Geometry check sheet. Reference: the model listing, model coordinates, mm. Round coordinates to 2 decimals unless told otherwise and drop trailing zeros. Write each loop counter-clockwise with the first axis right and the second up, starting at its lowest first coordinate (ties: lowest second). Pieces come first, ordered by that corner, then holes. Notation, with made-up numbers: (77, 61.25) -> (109, 61.25) arc R22 cw to (109, 68.25) -> close; hole circle Ø7 at (5, -22). An arc over 180 degrees is marked (long way). Use a Markdown table: item, result.
```python
from build123d import *

# Parameters (mm, degrees)
BOSS_EXTRUDE1_DEPTH = 6.35
CHAMFER1_SIZE       = 0.79375
SKETCH16_W          = 3.558466008
SKETCH16_H          = 3.18996611
CUT_EXTRUDE14_DEPTH = 208.663320883
SKETCH21_R          = 0.79375
CUT_EXTRUDE16_DEPTH = 3.175
LPATTERN3_COUNT     = 3
LPATTERN3_PITCH     = 2.032


# Read off the part's stored shape, not the designer's step: Boss-Extrude1
with BuildPart() as part:
    # Boss-Extrude1 outline → Boss-Extrude1 (new body)
    with BuildSketch(Plane.XY):
        with BuildLine():
            Line((22.436796564, 150), (19.069200519, 150))
            ThreePointArc((19.069200519, 150), (17.946668504, 150), (17.946668504, 151.122532015))
            Line((17.946668504, 151.122532015), (17.946668504, 158.877467985))
            ThreePointArc((17.946668504, 158.877467985), (17.946668504, 160), (19.069200519, 160))
            Line((19.069200519, 160), (22.436796564, 160))
            Line((22.436796564, 160), (22.436796564, 170))
            Line((22.436796564, 170), (19.069200519, 170))
            ThreePointArc((19.069200519, 170), (17.946668504, 170), (17.946668504, 171.122532015))
            Line((17.946668504, 171.122532015), (17.946668504, 178.877467985))
            ThreePointArc((17.946668504, 178.877467985), (17.946668504, 180), (19.069200519, 180))
            Line((19.069200519, 180), (22.436796564, 180))
            Line((22.436796564, 180), (22.436796564, 206.35))
            Line((22.436796564, 206.35), (17.436796564, 206.35))
            Line((17.436796564, 206.35), (17.436796564, 201.122532015))
            ThreePointArc((17.436796564, 201.122532015), (17.436796564, 200), (16.314264549, 200))
            Line((16.314264549, 200), (6.35, 200))
            Line((6.35, 200), (6.35, 191.122532015))
            ThreePointArc((6.35, 191.122532015), (6.35, 190), (5.227467985, 190))
            Line((5.227467985, 190), (0, 190))
            Line((0, 190), (0, 180))
            Line((0, 180), (5.227467985, 180))
            ThreePointArc((5.227467985, 180), (6.35, 180), (6.35, 178.877467985))
            Line((6.35, 178.877467985), (6.35, 171.122532015))
            ThreePointArc((6.35, 171.122532015), (6.35, 170), (5.227467985, 170))
            Line((5.227467985, 170), (0, 170))
            Line((0, 170), (0, 160))
            Line((0, 160), (5.227467985, 160))
            ThreePointArc((5.227467985, 160), (6.35, 160), (6.35, 158.877467985))
            Line((6.35, 158.877467985), (6.35, 151.122532015))
            ThreePointArc((6.35, 151.122532015), (6.35, 150), (5.227467985, 150))
            Line((5.227467985, 150), (0, 150))
            Line((0, 150), (0, 140))
            Line((0, 140), (5.227467985, 140))
            ThreePointArc((5.227467985, 140), (6.35, 140), (6.35, 138.877467985))
            Line((6.35, 138.877467985), (6.35, 131.122532015))
            ThreePointArc((6.35, 131.122532015), (6.35, 130), (5.227467985, 130))
            Line((5.227467985, 130), (0, 130))
            Line((0, 130), (0, 120))
            Line((0, 120), (5.227467985, 120))
            ThreePointArc((5.227467985, 120), (6.35, 120), (6.35, 118.877467985))
            Line((6.35, 118.877467985), (6.35, 111.122532015))
            ThreePointArc((6.35, 111.122532015), (6.35, 110), (5.227467985, 110))
            Line((5.227467985, 110), (0, 110))
            Line((0, 110), (0, 100))
            Line((0, 100), (5.227467985, 100))
            ThreePointArc((5.227467985, 100), (6.35, 100), (6.35, 98.877467985))
            Line((6.35, 98.877467985), (6.35, 91.122532015))
            ThreePointArc((6.35, 91.122532015), (6.35, 90), (5.227467985, 90))
            Line((5.227467985, 90), (0, 90))
            Line((0, 90), (0, 80))
            Line((0, 80), (5.227467985, 80))
            ThreePointArc((5.227467985, 80), (6.35, 80), (6.35, 78.877467985))
            Line((6.35, 78.877467985), (6.35, 71.122532015))
            ThreePointArc((6.35, 71.122532015), (6.35, 70), (5.227467985, 70))
            Line((5.227467985, 70), (0, 70))
            Line((0, 70), (0, 60))
            Line((0, 60), (5.227467985, 60))
            ThreePointArc((5.227467985, 60), (6.35, 60), (6.35, 58.877467985))
            Line((6.35, 58.877467985), (6.35, 51.122532015))
            ThreePointArc((6.35, 51.122532015), (6.35, 50), (5.227467985, 50))
            Line((5.227467985, 50), (0, 50))
            Line((0, 50), (0, 40))
            Line((0, 40), (5.227467985, 40))
            ThreePointArc((5.227467985, 40), (6.35, 40), (6.35, 38.877467985))
            Line((6.35, 38.877467985), (6.35, 31.122532015))
            ThreePointArc((6.35, 31.122532015), (6.35, 30), (5.227467985, 30))
            Line((5.227467985, 30), (0, 30))
            Line((0, 30), (0, 20))
            Line((0, 20), (5.227467985, 20))
            ThreePointArc((5.227467985, 20), (6.35, 20), (6.35, 18.877467985))
            Line((6.35, 18.877467985), (6.35, 11.122532015))
            ThreePointArc((6.35, 11.122532015), (6.35, 10), (5.227467985, 10))
            Line((5.227467985, 10), (0, 10))
            Line((0, 10), (0, 0))
            Line((0, 0), (16.314264549, 0))
            ThreePointArc((16.314264549, 0), (17.436796564, 0), (17.436796564, -1.122532015))
            Line((17.436796564, -1.122532015), (17.436796564, -6.35))
            Line((17.436796564, -6.35), (22.436796564, -6.35))
            Line((22.436796564, -6.35), (22.436796564, 10))
            Line((22.436796564, 10), (19.069200519, 10))
            ThreePointArc((19.069200519, 10), (17.946668504, 10), (17.946668504, 11.122532015))
            Line((17.946668504, 11.122532015), (17.946668504, 18.877467985))
            ThreePointArc((17.946668504, 18.877467985), (17.946668504, 20), (19.069200519, 20))
            Line((19.069200519, 20), (22.436796564, 20))
            Line((22.436796564, 20), (22.436796564, 30))
            Line((22.436796564, 30), (19.069200519, 30))
            ThreePointArc((19.069200519, 30), (17.946668504, 30), (17.946668504, 31.122532015))
            Line((17.946668504, 31.122532015), (17.946668504, 38.877467985))
            ThreePointArc((17.946668504, 38.877467985), (17.946668504, 40), (19.069200519, 40))
            Line((19.069200519, 40), (22.436796564, 40))
            Line((22.436796564, 40), (22.436796564, 50))
            Line((22.436796564, 50), (19.069200519, 50))
            ThreePointArc((19.069200519, 50), (17.946668504, 50), (17.946668504, 51.122532015))
            Line((17.946668504, 51.122532015), (17.946668504, 58.877467985))
            ThreePointArc((17.946668504, 58.877467985), (17.946668504, 60), (19.069200519, 60))
            Line((19.069200519, 60), (22.436796564, 60))
            Line((22.436796564, 60), (22.436796564, 70))
            Line((22.436796564, 70), (19.069200519, 70))
            ThreePointArc((19.069200519, 70), (17.946668504, 70), (17.946668504, 71.122532015))
            Line((17.946668504, 71.122532015), (17.946668504, 78.877467985))
            ThreePointArc((17.946668504, 78.877467985), (17.946668504, 80), (19.069200519, 80))
            Line((19.069200519, 80), (22.436796564, 80))
            Line((22.436796564, 80), (22.436796564, 90))
            Line((22.436796564, 90), (19.069200519, 90))
            ThreePointArc((19.069200519, 90), (17.946668504, 90), (17.946668504, 91.122532015))
            Line((17.946668504, 91.122532015), (17.946668504, 98.877467985))
            ThreePointArc((17.946668504, 98.877467985), (17.946668504, 100), (19.069200519, 100))
            Line((19.069200519, 100), (22.436796564, 100))
            Line((22.436796564, 100), (22.436796564, 110))
            Line((22.436796564, 110), (19.069200519, 110))
            ThreePointArc((19.069200519, 110), (17.946668504, 110), (17.946668504, 111.122532015))
            Line((17.946668504, 111.122532015), (17.946668504, 118.877467985))
            ThreePointArc((17.946668504, 118.877467985), (17.946668504, 120), (19.069200519, 120))
            Line((19.069200519, 120), (22.436796564, 120))
            Line((22.436796564, 120), (22.436796564, 130))
            Line((22.436796564, 130), (19.069200519, 130))
            ThreePointArc((19.069200519, 130), (17.946668504, 130), (17.946668504, 131.122532015))
            Line((17.946668504, 131.122532015), (17.946668504, 138.877467985))
            ThreePointArc((17.946668504, 138.877467985), (17.946668504, 140), (19.069200519, 140))
            Line((19.069200519, 140), (22.436796564, 140))
            Line((22.436796564, 140), (22.436796564, 150))
        make_face()
    extrude(amount=BOSS_EXTRUDE1_DEPTH)

    # Chamfer1
    chamfer1_edges = [part.edges().sort_by_distance(p)[0] for p in [
        (22.436796564, -6.35, 3.175),
        (17.436796564, -6.35, 3.175),
        (17.436796564, 206.35, 3.175),
        (22.436796564, 206.35, 3.175),
    ]]
    chamfer(chamfer1_edges, length=CHAMFER1_SIZE)

    # Sketch16 → Cut-Extrude14 (cut, through all)
    with BuildSketch(Plane.XZ):
        with Locations((13.17971111, 4.755016945)):
            Rectangle(SKETCH16_W, SKETCH16_H)
    extrude(amount=-CUT_EXTRUDE14_DEPTH, mode=Mode.SUBTRACT)

    # Sketch21 → Cut-Extrude16 (cut)
    with BuildSketch(Plane.XY.offset(6.35)):
        with Locations((20.404796564, 182.032)):
            Circle(SKETCH21_R)
    cut_extrude16 = extrude(amount=-CUT_EXTRUDE16_DEPTH, mode=Mode.SUBTRACT)

    # LPattern3: Cut-Extrude16 ×3
    with Locations(*[(0, i * LPATTERN3_PITCH, 0) for i in range(1, LPATTERN3_COUNT)]):
        add(cut_extrude16, mode=Mode.SUBTRACT)


solid = part.part
```
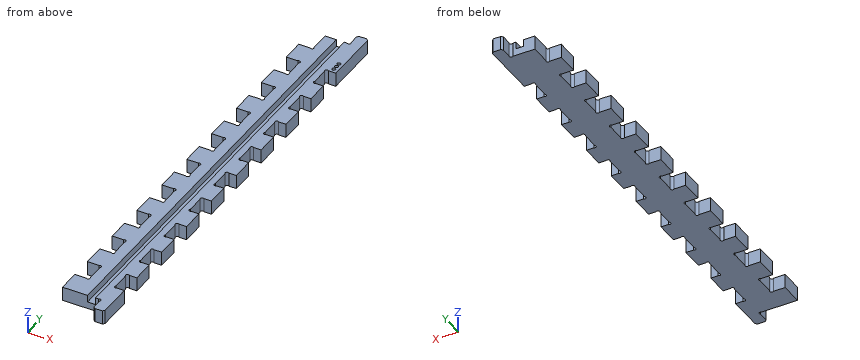
(1) Thickness scan on line 1 (X direction, y = 36, z = 4.5); line 2 (X direction, y = 189, z = 3.5); line 3 (Z direction, x = 14.5, y = 147). Record the ranges inside material, lowest first.
A:
| item | result |
|---|---|
| line 1 | x = 6.35 to 11.4, 14.96 to 17.95 |
| line 2 | x = 0 to 11.4, 14.96 to 22.44 |
| line 3 | z = 0 to 3.16 |
(2) Section check A-A on y = 137. Record the cut outline in (x, z), plus the area to 3 significant figures.
A:
| item | result |
|---|---|
| outline | (6.35, 0) -> (17.95, 0) -> (17.95, 6.35) -> (14.96, 6.35) -> (14.96, 3.16) -> (11.4, 3.16) -> (11.4, 6.35) -> (6.35, 6.35) -> close |
| area | 62.3 mm2 |
(3) Gauge pin test, flat ends, axial feed: pin 1 Ø0.8 at (x, y) = (20.5, 184) entering from +Z (3 decimals); pin 2 Ø2 at (y, z) = (154, 5.5) entering from -X; pin 3 Ø1.6 at (x, z) = (2.5, 4) entering from -Y. Record the tip position at first contact, or that the pin passes through.
A:
| item | result |
|---|---|
| pin 1 | stops at z = 3.175 |
| pin 2 | stops at x = 6.35 |
| pin 3 | stops at y = 0 |
(4) Section check B-B on z = 4.25. State how many separate pieces and enclosed holes the cut face has, plus the area to 3 significant figures.
A:
| item | result |
|---|---|
| separate pieces | 2 |
| enclosed holes | 3 |
| area | 2,780 mm2 |
